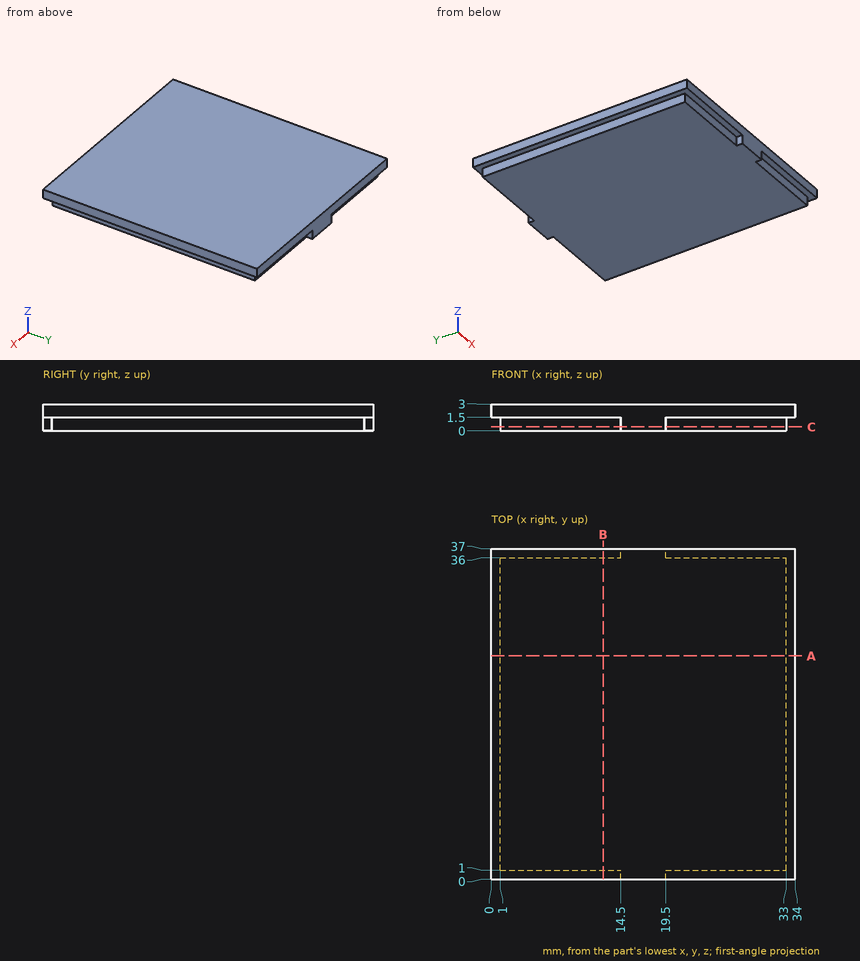
Print and shaded views of the part. All mm, measured from the part's lowest x, y and z. Give positions to 0.01 mm unless a question says otherwise; leave off trailing zeros. Order: outer loops, then holes, each group sorted by start corner. A loop starts at its lowest first (then second) coordinate and runs counter-clockwise, first axis right, second up. Notation, with made-up numbers: (-34, -1.5) -> (-4, -1.5) arc R13 cw to (-4, 21.5) -> close; hole circle Ø2 at (-26, 70). An arc over 180 degrees is marked (long way). Use CSV: the item, a comma, the result in double quotes.
1. Band-saw the part on B-B, the plane x = 12.5. Give the cut face in (y, z), then the cut area to 3 significant figures.
Outcome:
outline,"(0, 1.5) -> (1, 1.5) -> (1, 0) -> (36, 0) -> (36, 1.5) -> (37, 1.5) -> (37, 3) -> (0, 3) -> close"
area,"108 mm²"
2. Drill centre lines: line 1 along X through (y, z) = (25, 1.05); line 2 along Y through (x, z) = (12.5, 0.1). Where is each one in solid material? Low to high. Write a range as from..to.
Outcome:
line 1,"1..33"
line 2,"1..36"
3. Drop flat-ended pins along their axis: pin 1 (1.6 mm diameter, centred on x = 10, z = 0.5, fed in from -Y); pin 2 (0.8 mm diameter, centred on y = 15.5, z = 1, fed in from -X); pin 3 (0.8 mm diameter, centred on y = 36.5, z = 1, fed in from +X). Give the stop position or say it passes through.
Outcome:
pin 1,"y = 1"
pin 2,"x = 1"
pin 3,"x = 19.5"
4. Band-saw the part on A-A, the plane y = 25. Give the cut face in (x, z).
Outcome:
outline,"(0, 1.5) -> (1, 1.5) -> (1, 0) -> (33, 0) -> (33, 1.5) -> (34, 1.5) -> (34, 3) -> (0, 3) -> close"
5. Band-saw the part on C-C, the plane z = 0.45. Give the cut face in (x, y).
Outcome:
outline,"(1, 1) -> (14.5, 1) -> (14.5, 0) -> (19.5, 0) -> (19.5, 1) -> (33, 1) -> (33, 36) -> (19.5, 36) -> (19.5, 37) -> (14.5, 37) -> (14.5, 36) -> (1, 36) -> close"
